Check sheet for the drawn part. Datum: minimum x, y, z corner. Units: mm. A direction names the side the tool comes from. Round coordinates to 2 decimals unless told otherwise and drop trailing zeros. Write each loop counter-clockwise with the first axis right and the second up, starting at its lowest first coordinate (ties: lowest second). Pieces come first, ordered by that corner, then holes. Notation, with made-up numbers: (29.5, 60) -> (87.5, 60) arc R13 cw to (87.5, 84) -> close; hole circle Ø4 at (38.5, -39.5). An arc over 180 degrees is marked (long way). Use CSV: the item, a comma, the result in double quotes.
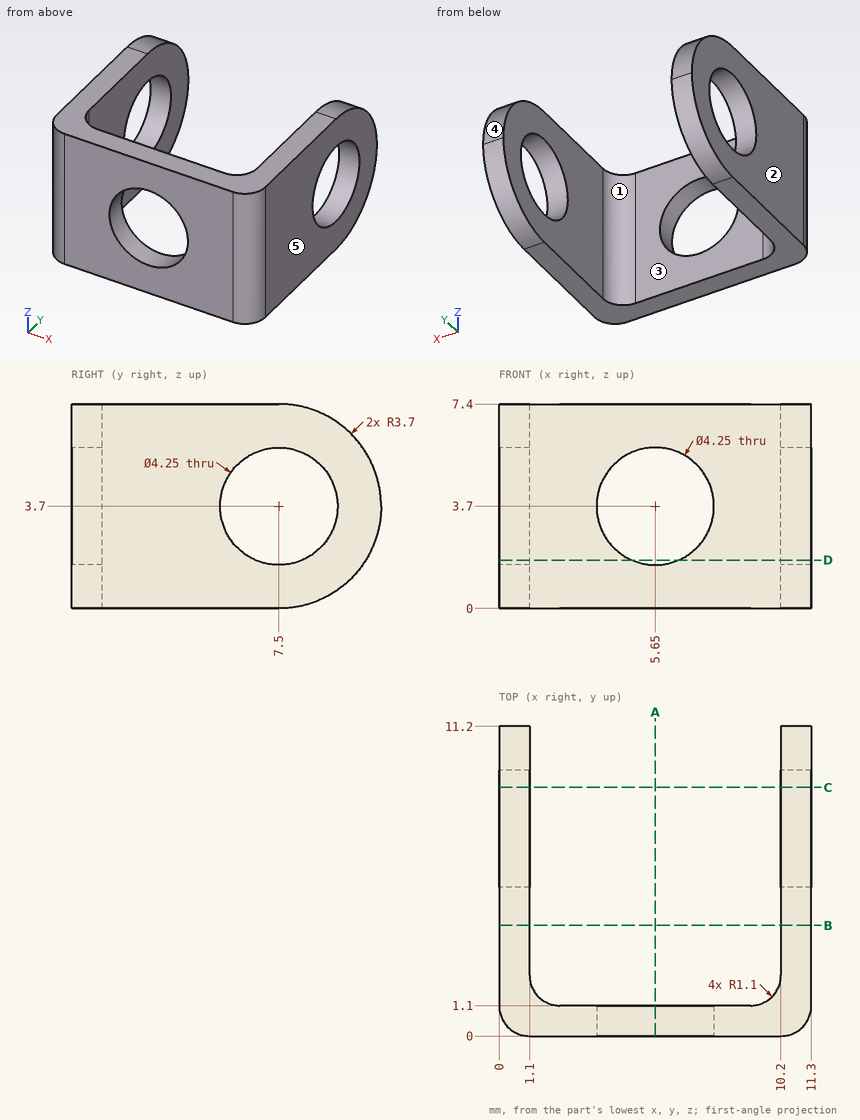
Q1. Go/stop test with a flat-tipped pin: P1, Ø2.5, axis at y = 7.5, z = 3.7, coming from the -X side. Record where the tip stops, or that it passes through.
Filled in:
P1,"through"
Q2. Mould release check, pull along X, two halves, no side actions. Record for the marked faces 3, 4 and 5: released by +X, released by -X, zero draft, split by the parting line, or undercut.
Filled in:
face 3,"undercut"
face 4,"zero draft"
face 5,"released by +X"
Q3. Material ranges on L1, parallel to Z at x = 5.65, y = 0.6 (1 decimal); L2, parallel to X at y = 6.5, z = 1.5; L3, parallel to Y at x = 7, z = 1, recorded low to high.
Filled in:
L1,"0 to 1.6, 5.8 to 7.4"
L2,"0 to 1.1, 10.2 to 11.3"
L3,"0 to 1.1"
Q4. Section check A-A (x = 5.65). Record the cut outline in (y, z) (1 decimal).
Filled in:
outline,"(0, 0) -> (1.1, 0) -> (1.1, 1.6) -> (0, 1.6) -> close; (0, 5.8) -> (1.1, 5.8) -> (1.1, 7.4) -> (0, 7.4) -> close"
Q5. Access from +Z, -Z, +X, -X, +Y, -Y to the whole of each face (thin tool, end or side, straight path). Record for the marked faces 1 and 2.
Filled in:
face 1,"+Z, -Z, +Y"
face 2,"+Z, -Z, -X, +Y, -Y"
Q6. Section check C-C (y = 9). Record the cut outline in (x, z) (1 decimal).
Filled in:
outline,"(0, 0.3) -> (1.1, 0.3) -> (1.1, 2.2) -> (0, 2.2) -> close; (0, 5.2) -> (1.1, 5.2) -> (1.1, 7.1) -> (0, 7.1) -> close; (10.2, 0.3) -> (11.3, 0.3) -> (11.3, 2.2) -> (10.2, 2.2) -> close; (10.2, 5.2) -> (11.3, 5.2) -> (11.3, 7.1) -> (10.2, 7.1) -> close"
Q7. Section check B-B (y = 4). Record the cut outline in (x, z).
Filled in:
outline,"(0, 0) -> (1.1, 0) -> (1.1, 7.4) -> (0, 7.4) -> close; (10.2, 0) -> (11.3, 0) -> (11.3, 7.4) -> (10.2, 7.4) -> close"
Q8. Section check D-D (z = 1.75). Record the cut outline in (x, y) (1 decimal).
Filled in:
outline,"(0, 1.1) arc R1.1 ccw to (1.1, 0) -> (4.8, 0) -> (4.8, 1.1) -> (2.2, 1.1) arc R1.1 cw to (1.1, 2.2) -> (1.1, 6.7) -> (0, 6.7) -> close; (0, 8.3) -> (1.1, 8.3) -> (1.1, 10.6) -> (0, 10.6) -> close; (6.5, 0) -> (10.2, 0) arc R1.1 ccw to (11.3, 1.1) -> (11.3, 6.7) -> (10.2, 6.7) -> (10.2, 2.2) arc R1.1 cw to (9.1, 1.1) -> (6.5, 1.1) -> close; (10.2, 8.3) -> (11.3, 8.3) -> (11.3, 10.6) -> (10.2, 10.6) -> close"
